Design review of the part built by this model. Coordinates are the model's own, in mm. A direction names the side the tool comes from. Coordinates: 2 decimals unless noted, no trailing zeros. Loops run counter-clockwise (first coordinate to the right, second up) from the corner with the lowest first, then second, coordinate; pieces in that order, holes last. Notation, with made-up numbers: M 20.5,61.25 L 36.5,61.25 A12 cw 36.5,82.25 Z; hole C 63,-34.75 d10. An arc over 180 degrees is marked long. Put each result on its own line as item: value. Start each with the question number.
(1) Take a section at A-A, the plane z = 31. Give the boundary of the cut face in (x, y) (3 decimals), then the cut area to 3 significant figures.
(2) Take a section at C-C, the plane y = -2.3. Give the boundary of the cut face in (x, z) (3 decimals).
(3) Clearance check with flat-ended pins moving along their axes: pin 1 (8 mm diameter, centred on x = 6.05, z = 28.58, fed in from -Y); pin 2 (1.6 mm diameter, centred on y = -1, z = 44, fed in from -X). State where each tip first meets the part, or that it passes through.
(4) The part is to be moulded in two halves that separate along X. For faces 3 (the flat face through (41, 0, 33)), 4 (the cylindrical face through (61.07, -1.57, 41.85)), 5 (the cylindrical face through (-3.995, -1.61, 35.176)), say which applies: +X half, -X half, draft (parallel to the pull), parting line (faces both ways), or undercut.
(5) For probe 1 along Z at (x, y) = (6.05, -1.45); probe 2 along X at (y, z) = (-1.35, 44); probe 3 along Z at (x, y) = (12, -1.25), list the stretches that pass through material, from the lowest coordinate up. Write a range as [from, to].
(6) For faces 1 (the flat face through (25, -2, 36.081)), 2 (the cylindrical face through (70.095, -1.61, 22.036)), list the 3-axis set-ups (+Z, -Z, +X, -X, +Y, -Y) from which the entire face can be reached by the end or side of a thin tool; tool diameter is ignored.
(7) Take a section at B-B, the plane x = 63.5. Give the boundary of the cut face in (y, z) (3 decimals), then the cut area to 3 significant figures.
(8) Take a section at D-D, the plane x = 32. Give the boundary of the cut face in (y, z) (3 decimals).
```python
from build123d import *

# Parameters (mm, degrees)
BOSS_EXTRUDE1_DEPTH  = 3.175
M8_CLEARANCE_HOLE1_D = 9
M6_CLEARANCE_HOLE1_D = 6.6
FILLET1_R            = 3.175


with BuildPart() as part:
    # Sketch1 → Boss-Extrude1 (new body)
    with BuildSketch(Plane(origin=(0, 0, 0), x_dir=(1, 0, 0), z_dir=(0, 1, 0))):
        Polygon((6.05, -36.0812086), (56, -36.0812086), (56, -44.0812086), (56, -51.0812086), (71, -51.0812086), (71, -44.0812086), (71, -21.0812086), (6.05, -21.0812086), (-4.95, -21.0812086), (-4.95, -36.0812086), align=None)
    extrude(amount=-BOSS_EXTRUDE1_DEPTH)

    # M8 Clearance Hole1 (through all)
    with Locations(Plane(origin=(0, -3.175, 0), x_dir=(-1, 0, 0), z_dir=(0, -1, 0))):
        with Locations((-6.05, -28.5812086)):
            Hole(M8_CLEARANCE_HOLE1_D / 2)

    # M6 Clearance Hole1 (through all)
    with Locations(Plane(origin=(0, -3.175, 0), x_dir=(-1, 0, 0), z_dir=(0, -1, 0))):
        with Locations((-63.5, -44.0812086)):
            Hole(M6_CLEARANCE_HOLE1_D / 2)

    # Fillet1
    fillet1_edges = [part.edges().sort_by_distance(p)[0] for p in [
        (71, -1.5875, 51.0812086),
        (56, -1.5875, 51.0812086),
        (56, -1.5875, 36.0812086),
        (-4.95, -1.5875, 36.0812086),
        (-4.95, -1.5875, 21.0812086),
        (71, -1.5875, 21.0812086),
    ]]
    fillet(fillet1_edges, radius=FILLET1_R)


solid = part.part
```
Computed values:
1. outline: M -4.95,-3.175 L 2.255,-3.175 L 2.255,0 L -4.95,0 Z; M 9.845,-3.175 L 71,-3.175 L 71,0 L 9.845,0 Z
1. area: 217 mm^2
2. outline: M -4.95,24.256 A3.175 ccw -1.775,21.081 L 67.825,21.081 A3.175 ccw 71,24.256 L 71,47.906 A3.175 ccw 67.825,51.081 L 59.175,51.081 A3.175 ccw 56,47.906 L 56,39.256 A3.175 cw 52.825,36.081 L -1.775,36.081 A3.175 ccw -4.95,32.906 Z; hole C 6.05,28.581 d9; hole C 63.5,44.081 d6.6
3. pin 1: passes through
3. pin 2: stops at x = 56
4. face 3: draft
4. face 4: undercut
4. face 5: -X half
5. probe 1: z = [21.08, 24.08], [33.08, 36.08]
5. probe 2: x = [56, 60.2], [66.8, 71]
5. probe 3: z = [21.08, 36.08]
6. face 1: +Z, -X, +Y, -Y
6. face 2: -Z, +X, +Y, -Y
7. outline: M -3.175,21.081 L 0,21.081 L 0,40.781 L -3.175,40.781 Z; M -3.175,47.381 L 0,47.381 L 0,51.081 L -3.175,51.081 Z
7. area: 74.3 mm^2
8. outline: M -3.175,21.081 L 0,21.081 L 0,36.081 L -3.175,36.081 Z
